Can you work these out from the model? Positions are in its coordinate system, mm. Coordinates: 2 decimals unless noted, no trailing zeros. Order: outer loops, then holes, each group sorted by start corner. A loop starts at its lowest first (then second) coordinate and runs counter-clockwise, first axis right, second up. Notation, with made-up numbers: (45, 62) -> (102, 62) arc R25 cw to (102, 96) -> close; hole circle Ø7 at (59, 18.25). An arc over 180 degrees is marked (long way). Answer in a Markdown table with one row per item. Add a question column.
1. Imagine slicing it at C-C on x = 4.25. Write out the boundary of the cut face in (y, z).
2. Imagine slicing it at A-A on x = 0. Write out the boundary of the cut face in (y, z).
3. If I drill on line 1 along Z through (x, y) = (0, 2.2); line 2 along X through (y, z) = (2.3, -85); line 3 along Z through (x, y) = (-1, 2.55), over which ranges is the centre line in solid material (lowest first)? Write a range as [from, to].
4. We'd pull the mould along X, two halves only. Please class faces 1 (the face through (0, 2, -90)), 2 (the face through (0, 5, -44)), 3 (the face through (0.4, 1.7, -83.4)): pulls with the +X half, pulls with the -X half, needs draft (parallel to the pull), parting line crosses it, or undercut.
5. Imagine slicing it at B-B on y = 2.25. Write out the boundary of the cut face in (x, z).
6. Will these pins go through, and if not, where does the flat tip stop? pin 1 (1.5 mm diameter, centred on x = 1.5, y = 2, fed in from -Z); pin 2 (4.5 mm diameter, centred on x = 0, z = -85, fed in from +Y).
Autodesk Inventor part; units mm, degrees
ref_plane "YZ Plane" through (0, 0, 0) normal (1, 0, 0) x (0, 1, 0)
ref_plane "XZ Plane" through (0, 0, 0) normal (0, 1, 0) x (-1, 0, 0)
ref_plane "XY Plane" through (0, 0, 0) normal (0, 0, 1) x (1, 0, 0)
sketch "Sketch1" plane through (0, 0, 0) normal (0, 1, 0) x (-1, 0, 0)
  line L0 (0, 0) -> (0, -90) construction
  line L1 (-5, -5) -> (-5, -85)
  line L2 (5, -85) -> (5, -5)
  arc A0 (5, -5) -> (-5, -5) centre (0, -5) ccw
  arc A1 (-5, -85) -> (5, -85) centre (0, -85) ccw
  circle A2 centre (0, -85) radius 1.65
  circle A3 centre (0, -5) radius 1.65
  point P0 (0, -45)
  dimension "d0" = 90
  dimension "d1" = 10
  dimension "d2" = 3.3
extrude "Extrusion1" add sketch "Sketch1" along normal blind 5
chamfer "Chamfer1" distance 1.5 angle 45 1 edges at (1.65, 5, -85)
properties part number "wiper_linkage_middle_arm" material "ABS Plastic"
Answers follow:
| question | item | result |
|---|---|---|
| 1 | outline | (0, -87.63) -> (5, -87.63) -> (5, -2.37) -> (0, -2.37) -> close |
| 2 | outline | (0, -90) -> (5, -90) -> (5, -88.15) -> (3.5, -86.65) -> (0, -86.65) -> close; (0, -83.35) -> (3.5, -83.35) -> (5, -81.85) -> (5, -6.65) -> (0, -6.65) -> close; (0, -3.35) -> (5, -3.35) -> (5, 0) -> (0, 0) -> close |
| 3 | line 1 | z = [-90, -86.65], [-83.35, -6.65], [-3.35, 0] |
| 3 | line 2 | x = [-5, -1.65], [1.65, 5] |
| 3 | line 3 | z = [-89.9, -86.31], [-83.69, -6.31], [-3.69, -0.1] |
| 4 | face 1 | parting line crosses it |
| 4 | face 2 | needs draft |
| 4 | face 3 | undercut |
| 5 | outline | (-5, -85) arc R5 ccw to (5, -85) -> (5, -5) arc R5 ccw to (-5, -5) -> close; hole circle Ø3.3 at (0, -85); hole circle Ø3.3 at (0, -5) |
| 6 | pin 1 | stops at z = -89.94 |
| 6 | pin 2 | stops at y = 4.1 |
